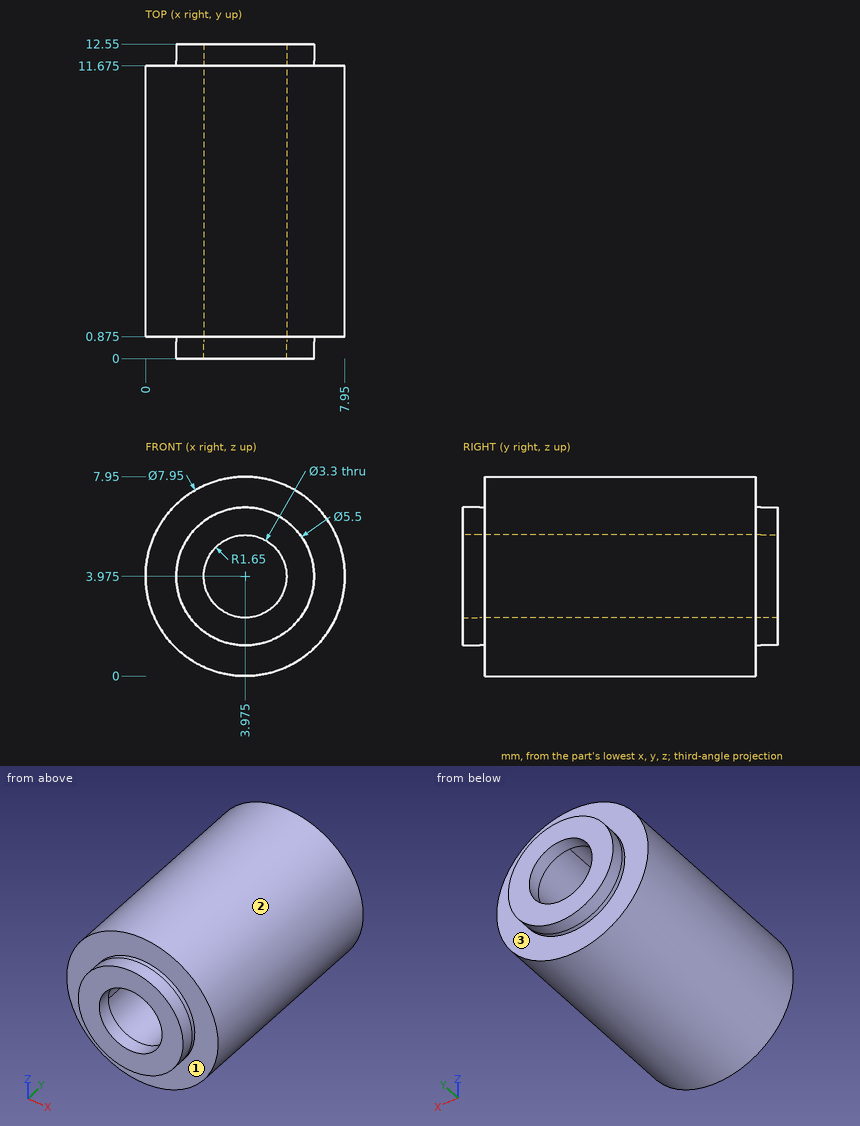
Print and shaded views of the part. All mm, measured from the part's lowest x, y and z. A direction names the side the tool comes from. Coordinates: 2 decimals unless noted, no trailing zeros.
Item 1: Tool access for the marked faces 1, 2 and 3: list every direction of +Z, -Z, +X, -X, +Y, -Y with a clear straight run to the whole face (end or side of a thin tool).
Filled in:
face 1: -Y
face 2: +Y, -Y
face 3: +Y
Item 2: Drill centre lines: L1, parallel to Y at x = 5, z = 7 (3 decimals); L2, parallel to Z at x = 4.25, y = 7; L3, parallel to Z at x = 3, y = 10.5 (1 decimal). Where is each one in solid material? Low to high.
Filled in:
L1: y = 0.875 to 11.675
L2: z = 0.01 to 2.35, 5.6 to 7.94
L3: z = 0.1 to 2.6, 5.3 to 7.8
Item 3: Drop flat-ended pins along their axis: pin 1 Ø1 at (y, z) = (5, 1) entering from +X (1 decimal); pin 2 Ø4.5 at (x, z) = (3.98, 3.98) entering from +Y; pin 3 Ø2 at (x, y) = (7, 10) entering from +Z. Give the stop position or say it passes through.
Filled in:
pin 1: stops at x = 7.1
pin 2: stops at y = 12.55
pin 3: stops at z = 7.4
